from build123d import *

# Parameters (mm, degrees)
F0_R      = 2.966363647
F1_DEPTH  = 15
F2_R      = 1.25
F3_DEPTH  = 15
F5_DEPTH  = 30
F7_DEPTH  = 25
F8_R      = 3
F9_R      = 3
F10_R     = 17.5
F11_DEPTH = 30
F12_R     = 3
F13_R     = 2


with BuildPart() as f1:
    # F0 (on Front) → F1 (new body, symmetric)
    with BuildSketch(Plane.XZ):
        with BuildLine():
            Line((-30, 0), (0, 0))
            Line((0, 0), (30, 0))
            Line((30, 0), (5, 130))
            ThreePointArc((5, 130), (0, 135), (-5, 130))
            Line((-5, 130), (-30, 0))
        make_face()
        with BuildLine():
            ThreePointArc((16.4291715262, 27.2951927036), (0, 10.8660211774), (-16.4291715262, 27.2951927036))
            Line((-16.4291715262, 27.2951927036), (-3.9969446867, 91.9427722692))
            ThreePointArc((-3.9969446867, 91.9427722692), (0, 95.9397169559), (3.9969446867, 91.9427722692))
            Line((3.9969446867, 91.9427722692), (16.4291715262, 27.2951927036))
        make_face(mode=Mode.SUBTRACT)
        with Locations((0, 130)):
            Circle(F0_R, mode=Mode.SUBTRACT)
    extrude(amount=F1_DEPTH, both=True)

    # F2 (on Top) → F3 (cut)
    with BuildSketch(Plane.XY):
        with Locations((-25, -10)):
            Circle(F2_R)
        with BuildLine():
            ThreePointArc((26.25, 10), (25, 11.25), (23.75, 10))
            ThreePointArc((23.75, 10), (25, 8.75), (26.25, 10))
        make_face()
        with Locations((-25, 10)):
            Circle(F2_R)
        with Locations((25, -10)):
            Circle(F2_R)
    extrude(amount=F3_DEPTH, mode=Mode.SUBTRACT)

    # F4 (on Right) → F5 (cut, symmetric)
    with BuildSketch(Plane.YZ):
        with BuildLine():
            Line((2.7910187355, 9.1569548885), (17.7158373854, 4.9780059552))
            Line((17.7158373854, 4.9780059552), (19.1600148357, 126.4660232181))
            Line((19.1600148357, 126.4660232181), (7.8171554744, 119.0036110992))
            ThreePointArc((7.8171554744, 119.0036110992), (-1.3503809801, 108.9970573428), (-4.6713938491, 95.8385727701))
            Line((-4.6713938491, 95.8385727701), (-4.6713938491, 21.9922982569))
            ThreePointArc((-4.6713938491, 21.9922982569), (-2.6702181322, 14.5687943509), (2.7910187355, 9.1569548885))
        make_face()
        with BuildLine():
            ThreePointArc((-9.9519597852, 95.8385729755), (-6.4277544412, 110.6791573106), (3.3923443925, 122.3508592262))
            Line((3.3923443925, 122.3508592262), (-9.9519597852, 122.5094883949))
            Line((-9.9519597852, 122.5094883949), (-9.9519597852, 95.8385729755))
        make_face()
    extrude(amount=F5_DEPTH, both=True, mode=Mode.SUBTRACT)

    # F6 (on Top) → F7 (cut)
    with BuildSketch(Plane.XY):
        with BuildLine():
            ThreePointArc((7.0281636992, -5.3187759427), (8.3555325008, -2.8052698872), (8.8138789708, 0))
            ThreePointArc((8.8138789708, 0), (-2.8052698872, 8.3555325008), (-7.0281636992, -5.3187759427))
            ThreePointArc((-7.0281636992, -5.3187759427), (0, -8.8138789708), (7.0281636992, -5.3187759427))
        make_face()
        with BuildLine():
            ThreePointArc((-7.0281636992, -5.3187759427), (-2.8052698872, 8.3555325008), (8.8138789708, 0))
            ThreePointArc((8.8138789708, 0), (8.3555325008, -2.8052698872), (7.0281636992, -5.3187759427))
            Line((7.0281636992, -5.3187759427), (22.7976655115, 15.5188456048))
            Line((22.7976655115, 15.5188456048), (0, 15.5188456048))
            Line((0, 15.5188456048), (-22.7976655115, 15.5188456048))
            Line((-22.7976655115, 15.5188456048), (-7.0281636992, -5.3187759427))
        make_face()
    extrude(amount=F7_DEPTH, mode=Mode.SUBTRACT)

    # F8
    f8_edges = [f1.edges().sort_by_distance(p)[0] for p in [
        (22.405013, 15, 2.86922),
    ]]
    fillet(f8_edges, radius=F8_R)

    # F9
    f9_edges = [f1.edges().sort_by_distance(p)[0] for p in [
        (-22.405013, 15, 2.86922),
        (-29.448227, 15, 2.86922),
        (29.448227, 15, 2.86922),
    ]]
    fillet(f9_edges, radius=F9_R)

    # F10 (on Top) → F11 (cut)
    with BuildSketch(Plane.XY):
        with Locations((0, 5.4938265468)):
            Circle(F10_R)
    extrude(amount=F11_DEPTH, mode=Mode.SUBTRACT)

    # F12
    f12_edges = [f1.edges().sort_by_distance(p)[0] for p in [
        (-17.284225, 8.233455, 3.816536),
        (17.284225, 8.233455, 3.816536),
    ]]
    fillet(f12_edges, radius=F12_R)

    # F13
    f13_edges = [f1.edges().sort_by_distance(p)[0] for p in [
        (-6.455736, -3.279808, 122.430174),
        (6.455736, -3.279808, 122.430174),
    ]]
    fillet(f13_edges, radius=F13_R)


solid = f1.part
Here's how the part is built. I have some questions about the finished solid (model axes, mm). A direction names the side the tool comes from. Round coordinates to 2 decimals unless told otherwise and drop trailing zeros. Loops run counter-clockwise (first coordinate to the right, second up) from the corner with the lowest first, then second, coordinate; pieces in that order, holes last. Notation, with made-up numbers: M 76,-25 L 99,-25 A24 ccw 99,-4 Z; hole C -35.5,27 d7. An arc over 180 degrees is marked long. Write each question's results on one line, items separated by ' | '. Start each with the question number.
(1) On a 3-axis mill with a long thin cutter (end or side, diameter ignored), from which of +Z, -Z, +X, -X, +Y, -Y can I reach the whole of each face in a straight line? I mean faces 5 (the flat face through (10.126, -9.908, 60.072)), 6 (the flat face through (15, -4.671, 59)), 7 (the cylindrical face through (5.592, -3.492, 123.178)). Say none if no direction works.
(2) Thinking about a two-plate mould opening in X: for faces 1 (the cylindrical face through (22.578, 14.695, 2.993)), 2 (the cylindrical face through (0, 0, 135)), 3 (the cylindrical face through (-25.27, 8.78, 3.73)), 4 (the flat face through (13, -15, 48)), which applies, pulls with the +X half, pulls with the -X half, needs draft (parallel to the pull), parting line crosses it, or undercut?
(3) I want a section at B-B (y = -7). State how many separate pieces and enclosed holes the cut face has, then the cut area to 3 significant figures.
(4) Will these pins go through, and if not, where does the flat tip stop? P1, Ø6, axis at y = -1, z = 86.5, coming from the +X side; P2, Ø2, axis at x = -25, y = -10, coming from the -Z side; P3, Ø3, axis at x = -25, y = 10, coming from the +Z side; P4, Ø6, axis at x = -17, z = 29.5, coming from the +Y side.
(5) If I drill on probe 1 along Y at (x, z) = (-25, 3.5); probe 2 along X at (y, z) = (10, 4); probe 3 along Z at (x, y) = (0, -5), over which ranges is the centre line in solid material (lowest first)? Write a range as from..to.
(6) I want a section at C-C (z = 113). Please give me the cut outline in (x, y).
(7) I want a section at A-A (z = 94). Please give me the cut outline in (x, y).
Solved:
1) face 5: +Y, -Y | face 6: +X, -X, +Y | face 7: +X
2) face 1: undercut | face 2: parting line crosses it | face 3: undercut | face 4: needs draft
3) separate pieces: 2 | enclosed holes: 1 | area: 2,280 mm²
4) P1: passes through | P2: stops at z = 15 | P3: stops at z = 7.56 | P4: stops at y = -4.67
5) probe 1: y = -15..-11.25, -8.75..8.75, 11.25..15 | probe 2: x = -29.23..-26.25, -23.75..-18.62, 18.62..23.75, 26.25..29.23 | probe 3: z = 95.94..113.23, 122.45..127.03, 132.97..135
6) outline: M -8.27,-15 L 8.27,-15 L 8.27,-9.95 L -8.27,-9.95 Z; M -8.27,-5.14 L 8.27,-5.14 L 8.27,1.28 L -8.27,1.28 Z
7) outline: M -11.92,-15 L -3.43,-15 L -3.43,-4.67 L -11.92,-4.67 Z; M 3.43,-15 L 11.92,-15 L 11.92,-4.67 L 3.43,-4.67 Z
